Input: part model. Units: mm. Frame: model coordinates. Face numbers are marked on the shaded views. A direction names the side the tool comes from. Coordinates: 2 decimals unless noted, no trailing zeros. Write each loop counter-clockwise with the first axis right and the second up, starting at its lowest first coordinate (ties: lowest second). Pieces come first, ordered by that corner, then holes.
1) Pin query (flat end, axial travel): pin 1 Ø4.5 at (x, z) = (16, 5) entering from +Y; pin 2 Ø0.8 at (y, z) = (32.5, 6.5) entering from -X; pin 3 Ø3 at (y, z) = (27, 4.5) entering from -X. Return the tip coordinate at first contact, or that it passes through.
2) Line query: L1, parallel to X at y = -9, z = 2.75; L2, parallel to Y at x = 40, z = 3; L3, parallel to Y at x = -29, z = 7.5. Output: solid intervals per line, ascending.
3) Section query B-B (z = 3.5). Output: boundary loops of the cut face in (x, y).
4) Section query D-D (x = -46.5). Output: boundary loops of the cut face in (y, z), then the cut area to 3 significant figures.
5) Set-up query: the marked faces 4, 5 and 6. Return all of +Z, -Z, +X, -X, +Y, -Y with unobstructed straight access to the full face (end or side cutting, diameter ignored); none if empty.
6) Draft query along Y for the marked faces 1, 2 and 3. Return one class per face: pulls with the +Y half, pulls with the -Y half, needs draft (parallel to the pull), parting line crosses it, or undercut.
7) Section query A-A (x = 11). Output: boundary loops of the cut face in (y, z).
8) Section query C-C (y = 41). Output: boundary loops of the cut face in (x, z), then the cut area to 3 significant figures.
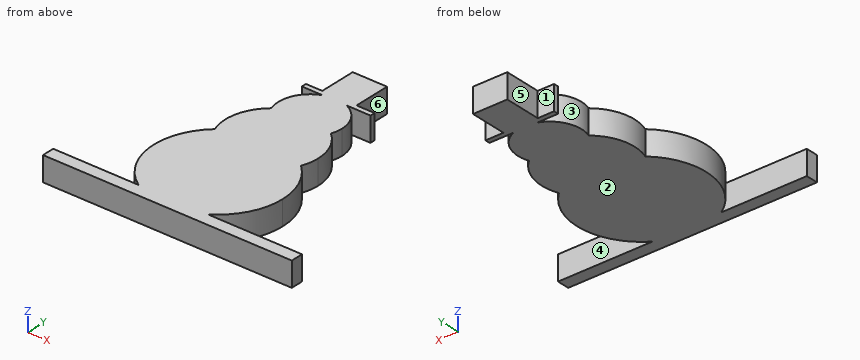
from build123d import *

# Parameters (mm, degrees)
F0_W     = 9.3442350626
F0_H     = 19.05
F0_W_2   = 8.4682106972
F1_DEPTH = 12.7


with BuildPart() as f1:
    # F0 (on Top) → F1 (new body)
    with BuildSketch(Plane.XY):
        with Locations((4.6721175313, 43.6261597422)):
            Rectangle(F0_W, F0_H)
        with Locations((-4.2341053486, 43.6261597422)):
            Rectangle(F0_W_2, F0_H)
        with BuildLine():
            Line((-16.9364213943, 31.5611597422), (-6.291250811, 31.5611597422))
            ThreePointArc((-6.291250811, 31.5611597422), (-3.2068706089, 32.4937729406), (0, 32.8086530862))
            Line((0, 32.8086530862), (0, 34.1011597422))
            Line((0, 34.1011597422), (-8.4682106972, 34.1011597422))
            Line((-8.4682106972, 34.1011597422), (-16.9364213943, 34.1011597422))
            Line((-16.9364213943, 34.1011597422), (-16.9364213943, 31.5611597422))
        make_face()
        with BuildLine():
            Line((0, 34.1011597422), (0, 32.8086530862))
            ThreePointArc((0, 32.8086530862), (3.2068706089, 32.4937729406), (6.291250811, 31.5611597422))
            Line((6.291250811, 31.5611597422), (18.6884663999, 31.5611597422))
            Line((18.6884663999, 31.5611597422), (18.6884663999, 34.1011597422))
            Line((18.6884663999, 34.1011597422), (9.3442350626, 34.1011597422))
            Line((9.3442350626, 34.1011597422), (0, 34.1011597422))
        make_face()
        with BuildLine():
            ThreePointArc((-6.291250811, 31.5611597422), (-15.090040572, 22.9640591319), (-15.4883746602, 10.6689312302))
            ThreePointArc((-15.4883746602, 10.6689312302), (0, 16.3211597422), (15.4883746602, 10.6689312302))
            ThreePointArc((15.4883746602, 10.6689312302), (16.2357924181, 13.4512326832), (16.4874933439, 16.3211597422))
            ThreePointArc((16.4874933439, 16.3211597422), (13.703364416, 25.4893242504), (6.291250811, 31.5611597422))
            Line((6.291250811, 31.5611597422), (0, 31.5611597422))
            Line((0, 31.5611597422), (-6.291250811, 31.5611597422))
        make_face()
        with BuildLine():
            ThreePointArc((-22.4394999049, -16.3700398839), (0, -7.7257658365), (22.4394999049, -16.3700398839))
            ThreePointArc((22.4394999049, -16.3700398839), (23.6416540668, -12.1219940808), (24.0469255787, -7.7257658365))
            ThreePointArc((24.0469255787, -7.7257658365), (21.8025505684, 2.4183663837), (15.4883746602, 10.6689312302))
            ThreePointArc((15.4883746602, 10.6689312302), (0, -0.1663336017), (-15.4883746602, 10.6689312302))
            ThreePointArc((-15.4883746602, 10.6689312302), (-23.2896416242, -1.7385108055), (-22.4394999049, -16.3700398839))
        make_face()
        with BuildLine():
            ThreePointArc((17.9249304532, -69.4115906954), (29.3109138189, -57.2848201084), (33.4472638545, -41.173029691))
            ThreePointArc((33.4472638545, -41.173029691), (30.5717135064, -27.605060328), (22.4394999049, -16.3700398839))
            ThreePointArc((22.4394999049, -16.3700398839), (0, -31.7726914152), (-22.4394999049, -16.3700398839))
            ThreePointArc((-22.4394999049, -16.3700398839), (-33.3267660846, -44.0095983393), (-17.9249304532, -69.4115906954))
            Line((-17.9249304532, -69.4115906954), (17.9249304532, -69.4115906954))
        make_face()
        with BuildLine():
            ThreePointArc((-22.4394999049, -16.3700398839), (0, -31.7726914152), (22.4394999049, -16.3700398839))
            ThreePointArc((22.4394999049, -16.3700398839), (0, -7.7257658365), (-22.4394999049, -16.3700398839))
        make_face()
        with BuildLine():
            ThreePointArc((15.4883746602, 10.6689312302), (0, 16.3211597422), (-15.4883746602, 10.6689312302))
            ThreePointArc((-15.4883746602, 10.6689312302), (0, -0.1663336017), (15.4883746602, 10.6689312302))
        make_face()
        with BuildLine():
            ThreePointArc((6.291250811, 31.5611597422), (3.2068706089, 32.4937729406), (0, 32.8086530862))
            Line((0, 32.8086530862), (0, 31.5611597422))
            Line((0, 31.5611597422), (6.291250811, 31.5611597422))
        make_face()
        with BuildLine():
            ThreePointArc((0, 32.8086530862), (-3.2068706089, 32.4937729406), (-6.291250811, 31.5611597422))
            Line((-6.291250811, 31.5611597422), (0, 31.5611597422))
            Line((0, 31.5611597422), (0, 32.8086530862))
        make_face()
        with BuildLine():
            Line((66.9182538986, -69.4115906954), (17.9249304532, -69.4115906954))
            ThreePointArc((17.9249304532, -69.4115906954), (0, -74.6202935455), (-17.9249304532, -69.4115906954))
            Line((-17.9249304532, -69.4115906954), (-62.283821404, -69.4115906954))
            Line((-62.283821404, -69.4115906954), (-62.283821404, -75.7877975702))
            Line((-62.283821404, -75.7877975702), (66.9182538986, -75.7877975702))
            Line((66.9182538986, -75.7877975702), (66.9182538986, -69.4115906954))
        make_face()
        with BuildLine():
            ThreePointArc((-17.9249304532, -69.4115906954), (0, -74.6202935455), (17.9249304532, -69.4115906954))
            Line((17.9249304532, -69.4115906954), (-17.9249304532, -69.4115906954))
        make_face()
    extrude(amount=F1_DEPTH)


solid = f1.part
Answer:
1. pin 1: stops at y = 34.1
1. pin 2: stops at x = -16.94
1. pin 3: stops at x = -13.7
2. L1: x = -24.01 to 24.01
2. L2: y = -75.79 to -69.41
2. L3: y = -75.79 to -69.41, -57.84 to -24.51
3. outline: (-62.28, -75.79) - (66.92, -75.79) - (66.92, -69.41) - (17.92, -69.41) arc R33.45 ccw to (22.44, -16.37) arc R24.05 ccw to (15.49, 10.67) arc R16.49 ccw to (6.29, 31.56) - (18.69, 31.56) - (18.69, 34.1) - (9.34, 34.1) - (9.34, 53.15) - (-8.47, 53.15) - (-8.47, 34.1) - (-16.94, 34.1) - (-16.94, 31.56) - (-6.29, 31.56) arc R16.49 ccw to (-15.49, 10.67) arc R24.05 ccw to (-22.44, -16.37) arc R33.45 ccw to (-17.92, -69.41) - (-62.28, -69.41) - close
4. outline: (-75.79, 0) - (-69.41, 0) - (-69.41, 12.7) - (-75.79, 12.7) - close
4. area: 81.0 mm2
5. face 4: +Z, -Z, +X
5. face 5: +Z, -Z, -X, +Y
5. face 6: +Z, -Z, +X, +Y
6. face 1: pulls with the +Y half
6. face 2: needs draft
6. face 3: undercut
7. outline: (-75.79, 0) - (28.6, 0) - (28.6, 12.7) - (-75.79, 12.7) - close; (31.56, 0) - (34.1, 0) - (34.1, 12.7) - (31.56, 12.7) - close
8. outline: (-8.47, 0) - (9.34, 0) - (9.34, 12.7) - (-8.47, 12.7) - close
8. area: 226 mm2
